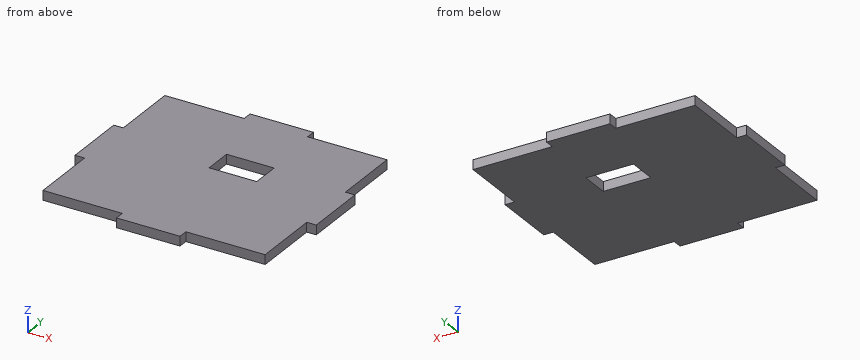
```python
from build123d import *

# Parameters (mm, degrees)
SKETCH1_W           = 70
SKETCH1_H           = 63
BOSS_EXTRUDE1_DEPTH = 3
SKETCH2_W           = 15
SKETCH2_H           = 9
CUT_EXTRUDE1_DEPTH  = 3
SKETCH4_W           = 3
SKETCH4_H           = 20
SKETCH4_W_2         = 20
SKETCH4_H_2         = 3
BOSS_EXTRUDE2_DEPTH = 3


with BuildPart() as part:
    # Sketch1 → Boss-Extrude1 (new body)
    with BuildSketch(Plane.XY):
        Rectangle(SKETCH1_W, SKETCH1_H)
    extrude(amount=BOSS_EXTRUDE1_DEPTH)

    # Sketch2 → Cut-Extrude1 (cut)
    with BuildSketch(Plane.XY.offset(3)):
        with Locations((4, 7.2)):
            Rectangle(SKETCH2_W, SKETCH2_H)
    extrude(amount=-CUT_EXTRUDE1_DEPTH, mode=Mode.SUBTRACT)

    # Sketch4 → Boss-Extrude2 (add)
    with BuildSketch(Plane.XY.offset(3)):
        with Locations((36.5, 0)):
            Rectangle(SKETCH4_W, SKETCH4_H)
        with Locations((-36.5, 0)):
            Rectangle(SKETCH4_W, SKETCH4_H)
        with Locations((0, 33)):
            Rectangle(SKETCH4_W_2, SKETCH4_H_2)
        with Locations((0, -33)):
            Rectangle(SKETCH4_W_2, SKETCH4_H_2)
    extrude(amount=-BOSS_EXTRUDE2_DEPTH)


solid = part.part
```
Source: CAD feature listing. Evaluate the final solid. Frame: model axes, mm. Round coordinates to 2 decimals unless told otherwise and drop trailing zeros. Loops run counter-clockwise (first coordinate to the right, second up) from the corner with the lowest first, then second, coordinate; pieces in that order, holes last. Notation, with made-up numbers: M 3.25,26.25 L 26.25,26.25 A16 ccw 26.25,47.25 Z; hole C -2.5,27 d6. An arc over 180 degrees is marked long. Use a Markdown table: item, result. Add a question column.
1. Cut plane A-A, the plane z = 1. Output: boundary loops of the cut face in (x, y).
2. Contact query for flat-ended pins moving along their axis: pin 1 (0.9 mm diameter, centred on x = 37, z = 2, fed in from +Y); pin 2 (0.9 mm diameter, centred on y = 21.5, z = 2, fed in from -X); pin 3 (1.5 mm diameter, centred on y = 33, z = 1, fed in from +X). Output: stop coordinate, or through.
3. Cut plane B-B, the plane x = -28. Output: boundary loops of the cut face in (y, z), and give its area (3 significant figures).
4. Ray query, line 1 along Y through (x, z) = (1, 1.35); line 2 along X through (y, z) = (3, 1.95); line 3 along X through (y, z) = (24, 1). Return the intervals inside material, ascending. Write a range as [from, to].
5. Cut plane C-C, the plane y = -24. Output: boundary loops of the cut face in (x, z), and give its area (3 significant figures).
Solution:
| question | item | result |
|---|---|---|
| 1 | outline | M -38,-10 L -35,-10 L -35,-31.5 L -10,-31.5 L -10,-34.5 L 10,-34.5 L 10,-31.5 L 35,-31.5 L 35,-10 L 38,-10 L 38,10 L 35,10 L 35,31.5 L 10,31.5 L 10,34.5 L -10,34.5 L -10,31.5 L -35,31.5 L -35,10 L -38,10 Z; hole M -3.5,2.7 L 11.5,2.7 L 11.5,11.7 L -3.5,11.7 Z |
| 2 | pin 1 | stops at y = 10 |
| 2 | pin 2 | stops at x = -35 |
| 2 | pin 3 | stops at x = 10 |
| 3 | outline | M -31.5,0 L 31.5,0 L 31.5,3 L -31.5,3 Z |
| 3 | area | 189 mm2 |
| 4 | line 1 | y = [-34.5, 2.7], [11.7, 34.5] |
| 4 | line 2 | x = [-38, -3.5], [11.5, 38] |
| 4 | line 3 | x = [-35, 35] |
| 5 | outline | M -35,0 L 35,0 L 35,3 L -35,3 Z |
| 5 | area | 210 mm2 |
